Geometry: final body of the model. Coordinates: model frame, mm. Round coordinates to 2 decimals unless told otherwise and drop trailing zeros. Write each loop counter-clockwise with the first axis right and the second up, starting at its lowest first coordinate (ties: lowest second). Pieces come first, ordered by that corner, then holes. Notation, with made-up numbers: M -29.5,-12.75 L -10.5,-12.75 A25 cw -10.5,25.25 Z; hole C -37.5,50 d3. An arc over 180 degrees is marked long. Put each result on its own line as item: value. Start each with the question number.
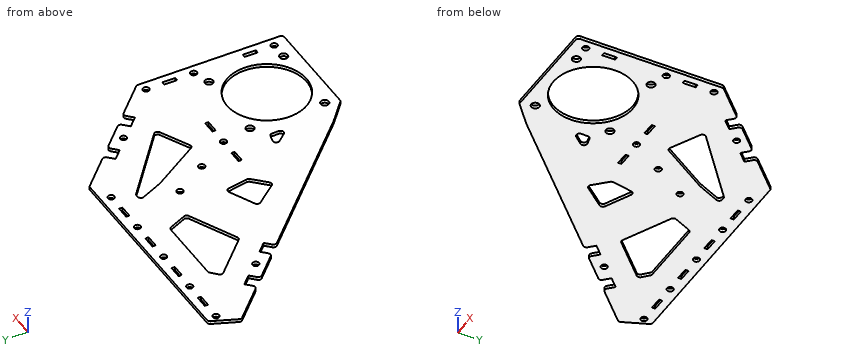
```python
from build123d import *

# Parameters (mm, degrees)
SKETCH_1_R      = 2
SKETCH_1_R_2    = 25
SKETCH_1_R_3    = 2.05
SKETCH_1_R_4    = 2.55
SKETCH_1_W      = 8.1
SKETCH_1_H      = 2.1
SKETCH_1_W_2    = 8.2
SKETCH_1_W_3    = 2.2
SKETCH_1_H_2    = 8.2
EXTRUDE_1_DEPTH = 2
FILLET_2_R      = 2


with BuildPart() as part:
    # 草图1 → 凸台-拉伸1 (new body)
    with BuildSketch(Plane.XY):
        Polygon((7.027428163, -4.999036262), (20.810808237, -16.956988843), (73.227648339, -16.964389058), (87.027428163, -16.964389058), (87.027428163, 75.054738201), (67.497807203, 94.584359161), (63.997628636, 91.084180595), (62.512704395, 89.599256354), (56.785139468, 95.326821282), (58.270063708, 96.811745522), (61.771734574, 100.31043179), (54.027428163, 108.054738201), (46.284614051, 115.797552313), (42.784435485, 112.297373746), (41.299511244, 110.812449505), (35.571946316, 116.540014433), (37.056870557, 118.024938674), (40.557049124, 121.52511724), (21.027428163, 141.054738201), (-114.884210676, 141.054738201), (-121.955278488, 123.983670389), (-100.755816342, 102.784208243), (-97.257364322, 106.282660262), (-95.772440082, 107.767584503), (-90.044875154, 102.040019575), (-91.529799395, 100.555095335), (-95.028251414, 97.056643315), (-87.28543216, 89.313824061), (-79.542612906, 81.571004807), (-76.044160887, 85.069456827), (-74.559236646, 86.554381067), (-68.831671719, 80.82681614), (-70.316595959, 79.341891899), (-73.815047978, 75.84343988), align=None)
        with Locations((-52.972571837, 135.054738201)):
            Circle(SKETCH_1_R, mode=Mode.SUBTRACT)
        with Locations((47.027428163, 15.054738201)):
            Circle(SKETCH_1_R_2, mode=Mode.SUBTRACT)
        with Locations(Location((-22.972571837, 135.054738201, 0), (0, 0, 180))):
            Circle(SKETCH_1_R, mode=Mode.SUBTRACT)
        with Locations((7.027428163, 135.054738201)):
            Circle(SKETCH_1_R, mode=Mode.SUBTRACT)
        with Locations(Location((-112.972571837, 135.054738201, 0), (0, 0, 180))):
            Circle(SKETCH_1_R, mode=Mode.SUBTRACT)
        with Locations((-82.972571837, 135.054738201)):
            Circle(SKETCH_1_R, mode=Mode.SUBTRACT)
        with Locations((49.784787476, 103.812097514)):
            Circle(SKETCH_1_R, mode=Mode.SUBTRACT)
        with Locations((-83.04451802, 93.554738201)):
            Circle(SKETCH_1_R, mode=Mode.SUBTRACT)
        with Locations((20.275835807, 57.054738201)):
            Circle(SKETCH_1_R_3, mode=Mode.SUBTRACT)
        with Locations((-6.58531727, 99.226748532)):
            Circle(SKETCH_1_R_3, mode=Mode.SUBTRACT)
        with Locations((70.527428163, -8.445261799)):
            Circle(SKETCH_1_R_4, mode=Mode.SUBTRACT)
        with Locations((23.527428163, -8.445261799)):
            Circle(SKETCH_1_R_4, mode=Mode.SUBTRACT)
        with Locations((23.527428163, 38.554738201)):
            Circle(SKETCH_1_R_4, mode=Mode.SUBTRACT)
        with Locations((70.527428163, 38.554738201)):
            Circle(SKETCH_1_R_4, mode=Mode.SUBTRACT)
        with Locations((81.392055944, 72.204829046)):
            Circle(SKETCH_1_R_3, mode=Mode.SUBTRACT)
        with Locations((81.392055944, -8.445261799)):
            Circle(SKETCH_1_R_3, mode=Mode.SUBTRACT)
        with Locations((81.392055944, 42.204829046)):
            Circle(SKETCH_1_R_3, mode=Mode.SUBTRACT)
        with Locations((6.845259268, 78.140743367)):
            Circle(SKETCH_1_R_3, mode=Mode.SUBTRACT)
        with Locations((-37.972571837, 135.054738201)):
            Rectangle(SKETCH_1_W, SKETCH_1_H, mode=Mode.SUBTRACT)
        with Locations((-7.972571837, 135.054738201)):
            Rectangle(SKETCH_1_W, SKETCH_1_H, mode=Mode.SUBTRACT)
        with Locations((-97.972571837, 135.054738201)):
            Rectangle(SKETCH_1_W, SKETCH_1_H, mode=Mode.SUBTRACT)
        with Locations((-67.972571837, 135.054738201)):
            Rectangle(SKETCH_1_W, SKETCH_1_H, mode=Mode.SUBTRACT)
        with Locations((5.275835807, 57.054738201)):
            Rectangle(SKETCH_1_W_2, SKETCH_1_H, mode=Mode.SUBTRACT)
        with Locations((35.275835807, 57.054738201)):
            Rectangle(SKETCH_1_W_2, SKETCH_1_H, mode=Mode.SUBTRACT)
        Polygon((-26.317798475, 106.3059132), (-58.783300448, 90.506724064), (-82.786741677, 114.510165293), (-76.96930946, 120.054738201), (-32.606331473, 120.054738201), align=None, mode=Mode.SUBTRACT)
        Polygon((47.299709176, 85.219712632), (24.92619293, 73.952191934), (4.862626833, 105.451990707), (-2.731253041, 122.054738201), (2.37892986, 122.054738201), align=None, mode=Mode.SUBTRACT)
        Polygon((-14.950211349, 60.939664471), (-17.845757969, 77.065019133), (-38.30861977, 67.106860342), (-24.982934729, 50.626518371), align=None, mode=Mode.SUBTRACT)
        Polygon((2.01437662, 34.262984309), (13.802642778, 20.368597473), (13.802642778, 31.594822975), align=None, mode=Mode.SUBTRACT)
        with Locations((81.392055944, 57.204829046)):
            Rectangle(SKETCH_1_W_3, SKETCH_1_H_2, mode=Mode.SUBTRACT)
        with Locations((81.392055944, 6.554738201)):
            Rectangle(SKETCH_1_W_3, SKETCH_1_H_2, mode=Mode.SUBTRACT)
    extrude(amount=EXTRUDE_1_DEPTH)

    # 圆角2
    fillet_2_edges = [part.edges().sort_by_distance(p)[0] for p in [
        (-26.317798475, 106.3059132, 1),
        (-32.606331473, 120.054738201, 1),
        (-76.96930946, 120.054738201, 1),
        (-82.786741677, 114.510165293, 1),
        (-58.783300448, 90.506724064, 1),
        (47.299709176, 85.219712632, 1),
        (2.37892986, 122.054738201, 1),
        (-2.731253041, 122.054738201, 1),
        (24.92619293, 73.952191934, 1),
        (-24.982934729, 50.626518371, 1),
        (-14.950211349, 60.939664471, 1),
        (-17.845757969, 77.065019133, 1),
        (-38.30861977, 67.106860342, 1),
        (13.802642778, 31.594822975, 1),
        (2.01437662, 34.262984309, 1),
        (13.802642778, 20.368597473, 1),
        (40.557049124, 121.52511724, 1),
        (46.284614051, 115.797552313, 1),
        (61.771734574, 100.31043179, 1),
        (67.497807203, 94.584359161, 1),
        (87.027428163, -16.964389058, 1),
        (-73.815047978, 75.84343988, 1),
        (-79.542612906, 81.571004807, 1),
        (-95.028251414, 97.056643315, 1),
        (-100.755816342, 102.784208243, 1),
        (-121.955278488, 123.983670389, 1),
        (-114.884210676, 141.054738201, 1),
    ]]
    fillet(fillet_2_edges, radius=FILLET_2_R)


solid = part.part
```
1) Section B-B, the plane y = 19.5. Output: boundary loops of the cut face in (x, z), and give its area (3 significant figures).
2) First-contact query: pin 1 (0.6 mm diameter, centred on x = 81, z = 1, fed in from +Y); pin 2 (0.6 mm diameter, centred on y = 57, z = 1.5, fed in from -X); pin 3 (1 mm diameter, centred on x = 36, z = 1.5, fed in from +Y). Flat tips, straight axial feed; report the tip coordinate or a pass-through.
3) Section C-C, the plane z = 1.15. Give the number of separate pieces and of enclosed holes in the cut face, and give its area (3 significant figures).
4) Section A-A, the plane x = 29. Output: boundary loops of the cut face in (y, z).
5) Ray query, probe 1 along Y at (x, z) = (-7, 1.7); probe 2 along Y at (x, z) = (38, 1.75); probe 3 along X at (y, z) = (110.5, 1.95). Return the intervals inside material, ascending.
Solved:
1. outline: M -17.47,0 L 22.43,0 L 22.43,2 L -17.47,2 Z; M 71.63,0 L 87.03,0 L 87.03,2 L 71.63,2 Z
1. area: 111 mm2
2. pin 1: stops at y = 81.38
2. pin 2: stops at x = -55.27
2. pin 3: stops at y = 126.58
3. separate pieces: 1
3. enclosed holes: 30
3. area: 16,000 mm2
4. outline: M -16.96,0 L -2.27,0 L -2.27,2 L -16.96,2 Z; M 32.38,0 L 76,0 L 76,2 L 32.38,2 Z; M 100.23,0 L 133.08,0 L 133.08,2 L 100.23,2 Z
5. probe 1: y = 9.03 to 97.22, 101.23 to 134, 136.1 to 141.05
5. probe 2: y = -16.96 to -8.26, 38.37 to 56, 58.1 to 80.54, 92.85 to 114.11, 118.97 to 124.08
5. probe 3: x = -108.47 to -78.78, -28.24 to 2.55, 16.47 to 51.58
